Here's how the part is built. I have some questions about the finished solid (model axes, mm). Coordinates: 2 decimals unless noted, no trailing zeros. Write each loop counter-clockwise with the first axis right and the second up, starting at its lowest first coordinate (ties: lowest second). Pieces come first, ordered by that corner, then holes. Notation, with made-up numbers: (67, 47.5) -> (97, 47.5) arc R17 cw to (97, 75.5) -> close; hole circle Ø3 at (71.25, 71). An arc over 180 degrees is marked (long way). Use a Markdown table: item, result. Add a question column.
Item 1: Imagine slicing it at B-B, the plane z = -8.5. Write out the boundary of the cut face in (x, y) (3 decimals).
Item 2: Imagine slicing it at D-D, the plane x = -37. Write out the boundary of the cut face in (y, z) (3 decimals), and give its area (3 significant figures).
Item 3: Will these pins go through, and if not, where does the flat tip stop? pin 1 Ø3 at (x, y) = (16.5, 2) entering from +Z; pin 2 Ø1 at (x, z) = (14, -6) entering from +Y.
Item 4: Imagine slicing it at C-C, the plane y = 2.7. Write out the boundary of the cut face in (x, z) (3 decimals), and give its area (3 significant figures).
Item 5: Imagine slicing it at A-A, the plane x = -12. Write out the boundary of the cut face in (y, z) (3 decimals).
Item 6: If I drill on line 1 along X through (y, z) = (1.45, 0); line 2 along Z through (x, y) = (-8.5, 4.55); line 3 along Z through (x, y) = (-19, 0.3), over which ranges is the centre line in solid material (lowest first)? Write a range as from..to.
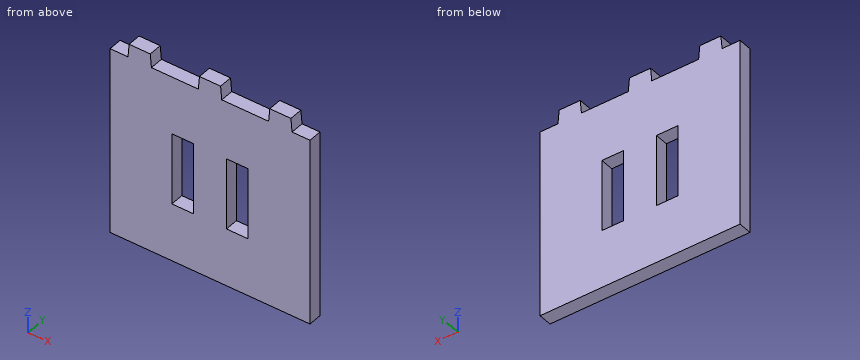
```python
from build123d import *

# Parameters (mm, degrees)
SKETCH2_W           = 85.279590556
SKETCH2_H           = 80
SKETCH2_W_2         = 9.25294304
SKETCH2_H_2         = 30.528437524
BOSS_EXTRUDE1_DEPTH = 5.715


with BuildPart() as part:
    # Sketch2 → Boss-Extrude1 (new body)
    with BuildSketch(Plane(origin=(0, 0, 0), x_dir=(1, 0, 0), z_dir=(0, 1, 0))):
        Rectangle(SKETCH2_W, SKETCH2_H)
        with Locations((-11.645107557, 0)):
            Rectangle(SKETCH2_W_2, SKETCH2_H_2, mode=Mode.SUBTRACT)
        with Locations((11.645107557, 0)):
            Rectangle(SKETCH2_W_2, SKETCH2_H_2, mode=Mode.SUBTRACT)
        Polygon((-25, -40), (-35, -40), (-34.5, -45.715), (-25.5, -45.715), align=None)
        Polygon((5, -40), (-5, -40), (-4.5, -45.715), (4.5, -45.715), align=None)
        Polygon((34.5, -45.715), (35, -40), (25, -40), (25.5, -45.715), align=None)
    extrude(amount=BOSS_EXTRUDE1_DEPTH)


solid = part.part
```
Ans:
| question | item | result |
|---|---|---|
| 1 | outline | (-42.64, 0) -> (-16.272, 0) -> (-16.272, 5.715) -> (-42.64, 5.715) -> close; (-7.019, 0) -> (7.019, 0) -> (7.019, 5.715) -> (-7.019, 5.715) -> close; (16.272, 0) -> (42.64, 0) -> (42.64, 5.715) -> (16.272, 5.715) -> close |
| 2 | outline | (0, -40) -> (5.715, -40) -> (5.715, 40) -> (0, 40) -> close |
| 2 | area | 457 mm^2 |
| 3 | pin 1 | stops at z = 40 |
| 3 | pin 2 | passes through |
| 4 | outline | (-42.64, -40) -> (42.64, -40) -> (42.64, 40) -> (35, 40) -> (34.5, 45.715) -> (25.5, 45.715) -> (25, 40) -> (5, 40) -> (4.5, 45.715) -> (-4.5, 45.715) -> (-5, 40) -> (-25, 40) -> (-25.5, 45.715) -> (-34.5, 45.715) -> (-35, 40) -> (-42.64, 40) -> close; hole (-16.272, -15.264) -> (-7.019, -15.264) -> (-7.019, 15.264) -> (-16.272, 15.264) -> close; hole (7.019, -15.264) -> (16.272, -15.264) -> (16.272, 15.264) -> (7.019, 15.264) -> close |
| 4 | area | 6,420 mm^2 |
| 5 | outline | (0, -40) -> (5.715, -40) -> (5.715, -15.264) -> (0, -15.264) -> close; (0, 15.264) -> (5.715, 15.264) -> (5.715, 40) -> (0, 40) -> close |
| 6 | line 1 | x = -42.64..-16.27, -7.02..7.02, 16.27..42.64 |
| 6 | line 2 | z = -40..-15.26, 15.26..40 |
| 6 | line 3 | z = -40..40 |
